Can you work these out from the model? Positions are in its coordinate system, mm. A direction names the side the tool comes from. Give positions to 0.01 mm unless a question says otherwise; leave off trailing zeros. Loops run counter-clockwise (first coordinate to the right, second up) from the corner with the lowest first, then second, coordinate; pieces in that order, holes last. Notation, with made-up numbers: M 74,16 L 94,16 A16 cw 94,23 Z; hole C 75,45 d11. An arc over 180 degrees is marked long. Put each result on its own line as item: value. Start each with the question number.
1) Imagine slicing it at A-A (y = 0). Write out the boundary of the cut face in (x, z).
2) Imagine slicing it at C-C (y = -19). Write out the boundary of the cut face in (x, z).
3) Imagine slicing it at D-D (z = -30). Write out the boundary of the cut face in (x, y).
4) For faces 1 (the cylindrical face through (180.155, 7.509, -23.846)), 2 (the flat face through (-22.8, -32.4, -0.1)), 3 (the flat face through (0, 1, -21)), 4 (the flat face through (0, 1, 22)), which set-ups out of +Z, -Z, +X, -X, +Y, -Y let a thin tool reach every point of the face, with its end or its side?
5) If we mould it in two halves opening along Z, with no side actions, what happens to faces 5 (the cylindrical face through (-69.994, 0.55, -0.14)), 6 (the flat face through (15, 0, 0)), 7 (the flat face through (-28, 1, 10))? For each: +Z half, -Z half, draft (parallel to the pull), parting line (faces both ways), or undercut.
6) Please list where these lines run through material, in increasing order: line 1 along Z through (x, y) = (160, 1.5); line 2 along Y through (x, z) = (141, 0); line 3 along X through (y, z) = (20, 2). Write a range as from..to.
7) For P1, Ø4, axis at x = 178.5, y = 12.5, coming from the +Z side; P2, Ø12, axis at x = 73.5, y = -23.5, coming from the -Z side; P3, Ø24, axis at y = -1, z = 29, coming from the -X side; P4, Ø8, axis at y = 22.5, z = 7.5, coming from the +X side, each with a flat end and sliding along its axis, tell me the tip position at first contact or that it passes through.
8) Imagine slicing it at B-B (x = 119). Write out the boundary of the cut face in (y, z).
from build123d import *

# Parameters (mm, degrees)
SKETCH1_R                = 40
BOSS_EXTRUDE1_DEPTH      = 350
SHELL1_T                 = -15
BOSS_EXTRUDE2_DEPTH      = 10
BOSS_EXTRUDE2_DEPTH_BACK = 10
SKETCH3_R                = 15
CUT_EXTRUDE1_START       = -68
SKETCH4_R                = 50.16795499
SKETCH4_R_2              = 40
CUT_EXTRUDE1_DEPTH       = 68


with BuildPart() as part:
    # Sketch1 → Boss-Extrude1 (new body)
    with BuildSketch(Plane(origin=(0, 0, 0), x_dir=(0, 0, -1), z_dir=(1, 0, 0))):
        Circle(SKETCH1_R)
    extrude(amount=BOSS_EXTRUDE1_DEPTH)

    # Shell1
    shell1_openings = [part.faces().sort_by_distance(p)[0] for p in [
        (350, 0, 0),
    ]]
    offset(amount=SHELL1_T, openings=shell1_openings, kind=Kind.INTERSECTION)

    # Sketch3 → Boss-Extrude2 (add, two sides: drawn at the far end of the back side and taken through both)
    with BuildSketch(Plane.XY.offset(-BOSS_EXTRUDE2_DEPTH_BACK)):
        with BuildLine():
            Line((0, 40), (-45, 25))
            ThreePointArc((-45, 25), (-70, 0), (-45, -25))
            Line((-45, -25), (0, -40))
            Line((0, -40), (0, 40))
        make_face()
        with Locations((-45, 0)):
            Circle(SKETCH3_R, mode=Mode.SUBTRACT)
    extrude(amount=BOSS_EXTRUDE2_DEPTH + BOSS_EXTRUDE2_DEPTH_BACK)

    # Sketch4 → Cut-Extrude1 (cut)
    with BuildSketch(Plane(origin=(0, 0, 0), x_dir=(0, 0, -1), z_dir=(1, 0, 0)).offset(CUT_EXTRUDE1_START)):
        Circle(SKETCH4_R)
        with Locations(Location((0, 0, 0), (0, 0, 255.522487814))):
            Circle(SKETCH4_R_2, mode=Mode.SUBTRACT)
    extrude(amount=CUT_EXTRUDE1_DEPTH, mode=Mode.SUBTRACT)


solid = part.part
Recorded:
1. outline: M -70,-10 L -60,-10 L -60,10 L -70,10 Z; M -30,-10 L 0,-10 L 0,-40 L 350,-40 L 350,-25 L 15,-25 L 15,25 L 350,25 L 350,40 L 0,40 L 0,10 L -30,10 Z
2. outline: M -61.25,-10 L 0,-10 L 0,-35.2 L 350,-35.2 L 350,-16.25 L 15,-16.25 L 15,16.25 L 350,16.25 L 350,35.2 L 0,35.2 L 0,10 L -61.25,10 Z
3. outline: M 0,-26.46 L 350,-26.46 L 350,26.46 L 0,26.46 Z
4. face 1: +X
4. face 2: +Z, -Z, -X, -Y
4. face 3: -Z, -X, +Y, -Y
4. face 4: +Z, -X, +Y, -Y
5. face 5: draft
5. face 6: undercut
5. face 7: +Z half
6. line 1: -39.97..-24.95, 24.95..39.97
6. line 2: -40..-25, 25..40
6. line 3: -60..15
7. P1: z = 38.6
7. P2: z = -35.97
7. P3: x = 0
7. P4: x = 350
8. outline: C 0,0 d80; hole C 0,0 d50
